Source: CAD feature listing. Evaluate the final solid. Frame: model axes, mm. Round coordinates to 2 decimals unless told otherwise and drop trailing zeros. Write each loop counter-clockwise with the first axis right and the second up, starting at its lowest first coordinate (ties: lowest second). Pieces come first, ordered by that corner, then holes. Notation, with made-up numbers: (67.25, -9.5) - (116.25, -9.5) arc R17 ccw to (116.25, 5.5) - close; hole circle Ø7 at (-34, -24.5). An arc over 180 degrees is marked (long way). Write item = value, one per line. Start each with the question number.
```python
from build123d import *

# Parameters (mm, degrees)
SKETCH_2_R      = 8
SKETCH_2_R_2    = 13
EXTRUDE_1_DEPTH = 30


with BuildPart() as part:
    # Эскиз2 → Бобышка-Вытянуть1 (new, symmetric)
    with BuildSketch(Plane.XY):
        with BuildLine():
            Line((14.78207252, -35.687079958), (58.040092118, -140.121177553))
            ThreePointArc((58.040092118, -140.121177553), (58.040092118, -155.428514848), (47.216170115, -166.252436851))
            Line((47.216170115, -166.252436851), (0, -185.810014876))
            Line((0, -185.810014876), (-47.216170115, -166.252436851))
            ThreePointArc((-47.216170115, -166.252436851), (-58.040092118, -155.428514848), (-58.040092118, -140.121177553))
            Line((-58.040092118, -140.121177553), (-14.78207252, -35.687079958))
            ThreePointArc((-14.78207252, -35.687079958), (0, -25.810014876), (14.78207252, -35.687079958))
        make_face()
        with Locations((0, -41.810014876)):
            Circle(SKETCH_2_R, mode=Mode.SUBTRACT)
        with Locations((0, -161.810014876)):
            Circle(SKETCH_2_R_2, mode=Mode.SUBTRACT)
    extrude(amount=EXTRUDE_1_DEPTH, both=True)


solid = part.part
```
(1) Ray query, L1, parallel to Y at x = 0, z = 12.5; L2, parallel to X at y = -113.5, z = 1.5; L3, parallel to Y at x = 18, z = 11. Return the intervals inside material, ascending. Write a range as from..to.
(2) Section A-A (y = -164). Return the cut outline in (x, z), plus the area to 3 significant figures.
(3) Section D-D (x = -33). Return the cut outline in (y, z).
(4) Section B-B (x = 3). Return the cut outline in (y, z), plus the area to 3 significant figures.
(5) Section C-C (z = 2.5). Return the cut outline in (x, y), plus the area to 3 significant figures.
(6) Contact query for flat-ended pins moving along their axis: P1, Ø2, axis at y = -166, z = -2, coming from the -X side; P2, Ø1.5, axis at y = -118, z = -3, coming from the +X side; P3, Ø1.5, axis at y = -129, z = 19, coming from the +X side. Output: stop coordinate, or through.
(7) Pull-direction query (X, two-part tool) for faces 1 (the flat face through (23.939, -175.894, 0.42)), 2 (the flat face through (1, -122, 30)), 3 (the flat face through (-36.7, -88.6, 0.4)), 4 (the cylindrical face through (-1.69, -148.92, -0.42)); classes: +X half, -X half, draft (parallel to the pull), parting line (faces both ways), or undercut.
Solution:
q1.L1 = -185.81..-174.81, -148.81..-49.81, -33.81..-25.81
q1.L2 = -47.01..47.01
q1.L3 = -178.35..-43.46
q2.outline = (-51.26, -30) - (-12.81, -30) - (-12.81, 30) - (-51.26, 30) - close; (12.81, -30) - (51.26, -30) - (51.26, 30) - (12.81, 30) - close
q2.area = 4,610 mm^2
q3.outline = (-172.14, -30) - (-79.67, -30) - (-79.67, 30) - (-172.14, 30) - close
q4.outline = (-184.57, -30) - (-174.46, -30) - (-174.46, 30) - (-184.57, 30) - close; (-149.16, -30) - (-49.23, -30) - (-49.23, 30) - (-149.16, 30) - close; (-34.39, -30) - (-26.09, -30) - (-26.09, 30) - (-34.39, 30) - close
q4.area = 7,100 mm^2
q5.outline = (-58.04, -140.12) arc R20 ccw to (-47.22, -166.25) - (0, -185.81) - (47.22, -166.25) arc R20 ccw to (58.04, -140.12) - (14.78, -35.69) arc R16 ccw to (-14.78, -35.69) - close; hole circle Ø26 at (0, -161.81); hole circle Ø16 at (0, -41.81)
q5.area = 11,000 mm^2
q6.P1 = -49.73
q6.P2 = 49.19
q6.P3 = 53.74
q7.face_1 = +X half
q7.face_2 = draft
q7.face_3 = -X half
q7.face_4 = undercut
